```python
from build123d import *

# Parameters (mm, degrees)
SKETCH1_R               = 88
SKETCH1_R_2             = 85
BOSS_EXTRUDE1_DEPTH     = 360
CUT_EXTRUDE1_REACH      = 412.268
CUT_EXTRUDE1_END_RADIUS = 85
SKETCH2_R               = 2.75


with BuildPart() as part:
    # Sketch1 → Boss-Extrude1 (new body)
    with BuildSketch(Plane(origin=(0, 0, 0), x_dir=(1, 0, 0), z_dir=(0, 1, 0))):
        with Locations(Location((0, 0, 0), (0, 0, 90))):
            Circle(SKETCH1_R)
        with Locations(Location((0, 0, 0), (0, 0, 90))):
            Circle(SKETCH1_R_2, mode=Mode.SUBTRACT)
    extrude(amount=BOSS_EXTRUDE1_DEPTH)

    # Cut-Extrude1: up to this cylinder (the profile starts outside it)
    cut_extrude1_end = Plane(origin=(0, 35, 0), z_dir=(0, -1, 0)) * Cylinder(CUT_EXTRUDE1_END_RADIUS, 995.536, mode=Mode.PRIVATE)
    # Sketch2 → Cut-Extrude1 (cut, up to the surface)
    with BuildSketch(Plane.ZY.offset(88), mode=Mode.PRIVATE) as cut_extrude1_sk1:
        with Locations((0, 35)):
            Circle(SKETCH2_R)
    cut_extrude1_tool1 = extrude(cut_extrude1_sk1.sketch, amount=-CUT_EXTRUDE1_REACH, mode=Mode.PRIVATE) - cut_extrude1_end
    add(cut_extrude1_tool1.solids().sort_by_distance((-88, 35, 0))[0], mode=Mode.SUBTRACT)

    # Sketch4 → Cut-Revolve1 (revolve, cut)
    with BuildSketch(Plane.XZ.offset(-35), mode=Mode.PRIVATE) as cut_revolve1_sk:
        Polygon((-88, 0), (-88, -5), (-83, 0), align=None)
    revolve(cut_revolve1_sk.sketch.rotate(Axis((-88, 35, 0), (1, 0, 0)), 180), axis=Axis((-88, 35, 0), (1, 0, 0)), mode=Mode.SUBTRACT)


solid = part.part
```
Could you check a few things on this model? Use its own coordinates, in mm. Round coordinates to 2 decimals unless told otherwise and drop trailing zeros. Loops run counter-clockwise (first coordinate to the right, second up) from the corner with the lowest first, then second, coordinate; pieces in that order, holes last. Notation, with made-up numbers: (-34.5, 9) -> (15.5, 9) arc R10 ccw to (15.5, 28) -> close; hole circle Ø7 at (9.5, 41.5). An arc over 180 degrees is marked (long way). One line per question, with ' | ' between items.
(1) If we section it at C-C on y = 71: List the corners of the cut face in (x, z) for me.
Model answer:
outline: circle Ø176 at (0, 0); hole circle Ø170 at (0, 0)
(2) If we section it at B-B on z = 77: List the corners of the cut face in (x, y) for me, and give its area (3 significant figures).
Model answer:
outline: (-42.6, 0) -> (-36, 0) -> (-36, 360) -> (-42.6, 360) -> close; (36, 0) -> (42.6, 0) -> (42.6, 360) -> (36, 360) -> close | area: 4,750 mm^2
(3) If I drill on probe 1 along X at (y, z) = (175, -3.5); probe 2 along Y at (x, z) = (-85.1, 0); probe 3 along Z at (x, y) = (-2, 274.5), over which ranges is the centre line in solid material (lowest first)?
Model answer:
probe 1: x = -87.93 to -84.93, 84.93 to 87.93 | probe 2: y = 0 to 32.25, 37.75 to 360 | probe 3: z = -87.98 to -84.98, 84.98 to 87.98
(4) Thinking about a two-plate mould opening in Z: for faces 1 (the face through (-46, 0, 72)), 2 (the face through (-85.86, 37.79, -0.62)), 3 (the face through (85.907, 177.48, 19.077)), which applies, released by +Z, released by -Z, zero draft, split by the parting line, or undercut?
Model answer:
face 1: zero draft | face 2: undercut | face 3: split by the parting line
(5) If we section it at A-A on x = 0: List the corners of the cut face in (y, z) for me, and give its area (3 significant figures).
Model answer:
outline: (0, -88) -> (360, -88) -> (360, -85) -> (0, -85) -> close; (0, 85) -> (360, 85) -> (360, 88) -> (0, 88) -> close | area: 2,160 mm^2
(6) For pin 1 Ø4 at (x, y) = (-23.5, 181.5) entering from -Z; pin 2 Ø6 at (y, z) = (159, 2.5) entering from -X; pin 3 Ø4 at (x, y) = (-67, 319) entering from +Z, each with a flat end and sliding along its axis, tell me the tip position at first contact or that it passes through.
Model answer:
pin 1: stops at z = -85.33 | pin 2: stops at x = -88 | pin 3: stops at z = 59.32
